```python
from build123d import *

# Parameters (mm, degrees)
F1_DEPTH = 101.6
F3_DEPTH = 25.4


with BuildPart() as f1:
    # F0 (on Front) → F1 (new body)
    with BuildSketch(Plane.XZ):
        Polygon((-38.1, 0), (0, 0), (0, 101.6), (-25.391597, 101.6), (-25.391597, 50.8), (-76.191597, 50.8), (-76.191597, 63.5), (-101.6, 63.5), (-101.6, 0), (-63.5, 0), (-63.5, 25.4), (-38.1, 25.4), align=None)
    extrude(amount=F1_DEPTH)

    # F2 (on face) → F3 (cut)
    with BuildSketch(Plane.YZ):
        Polygon((-101.6, 101.6), (-101.6, 50.8), (-50.8, 101.6), align=None)
    extrude(amount=-F3_DEPTH, mode=Mode.SUBTRACT)


solid = f1.part
```
Input: part model. Units: mm. Frame: model coordinates. A direction names the side the tool comes from. Give positions to 0.01 mm unless a question says otherwise; leave off trailing zeros. Write each loop counter-clockwise with the first axis right and the second up, starting at its lowest first coordinate (ties: lowest second). Pieces come first, ordered by that corner, then holes. Notation, with made-up numbers: (64.5, 34) - (69.5, 34) arc R23 ccw to (69.5, 67) - close; hole circle Ø1 at (4.5, 58). An arc over 180 degrees is marked (long way). Write item = value, one per line. Start each with the question number.
1) Cut plane C-C (z = 20.5). Return loops of the section in (x, y), and give its area (3 significant figures).
2) Cut plane D-D (x = -54). Return loops of the section in (y, z).
3) Material intervals for L1, parallel to X at y = -69, z = 22.5; L2, parallel to X at y = -6, z = 55; L3, parallel to X at y = -67.5, z = 72, sorted ascending. Write a range as [from, to].
4) Reachability of faces 1 (the face through (-89, -50, 63.5)), 2 (the face through (-25.392, -39, 77)), 3 (the face through (-38.1, -50, 13)) from +Z, -Z, +X, -X, +Y, -Y: full face, straight path, thin tool, end or side. Return the list, or none.
5) Cut plane A-A (z = 57). Return loops of the section in (x, y).
6) Pin query (flat end, axial travel): pin 1 (12.5 mm diameter, centred on x = -83.5, y = -28, fed in from +Z); pin 2 (1 mm diameter, centred on x = -48, y = -10.5, fed in from -Z); pin 3 (4 mm diameter, centred on y = -60, z = 79.5, fed in from -X). Return the tip coordinate at first contact, or that it passes through.
7) Cut plane B-B (y = -54). Return loops of the section in (x, z).
8) Draft query along X for faces 4 (the face through (0, -50, 50)), 5 (the face through (-13, -25, 101.6)), 6 (the face through (-51, -50, 25.4)). Return one class per face: pulls with the +X half, pulls with the -X half, needs draft (parallel to the pull), parting line crosses it, or undercut.
Answers follow:
q1.outline = (-101.6, -101.6) - (-63.5, -101.6) - (-63.5, 0) - (-101.6, 0) - close; (-38.1, -101.6) - (0, -101.6) - (0, 0) - (-38.1, 0) - close
q1.area = 7,740 mm^2
q2.outline = (-101.6, 25.4) - (0, 25.4) - (0, 50.8) - (-101.6, 50.8) - close
q3.L1 = [-101.6, -63.5], [-38.1, 0]
q3.L2 = [-101.6, -76.19], [-25.39, 0]
q3.L3 = [-25.39, 0]
q4.face_1 = +Z, -X, +Y, -Y
q4.face_2 = +Z, +Y, -Y
q4.face_3 = -Z, +Y, -Y
q5.outline = (-101.6, -101.6) - (-76.19, -101.6) - (-76.19, 0) - (-101.6, 0) - close; (-25.39, -95.4) - (0, -95.4) - (0, 0) - (-25.39, 0) - close
q6.pin_1 = 63.5
q6.pin_2 = 25.4
q6.pin_3 = -25.39
q7.outline = (-101.6, 0) - (-63.5, 0) - (-63.5, 25.4) - (-38.1, 25.4) - (-38.1, 0) - (0, 0) - (0, 98.4) - (-25.39, 98.4) - (-25.39, 50.8) - (-76.19, 50.8) - (-76.19, 63.5) - (-101.6, 63.5) - close
q8.face_4 = pulls with the +X half
q8.face_5 = needs draft
q8.face_6 = undercut
